Here's how the part is built. I have some questions about the finished solid (model axes, mm). Face numbers are marked on the shaded views. A direction names the side the tool comes from. Coordinates: 2 decimals unless noted, no trailing zeros. Order: outer loops, then holes, each group sorted by start corner. A loop starts at its lowest first (then second) coordinate and runs counter-clockwise, first axis right, second up. Notation, with made-up numbers: (84.5, 77.25) - (124.5, 77.25) arc R23 ccw to (124.5, 98.25) - close; hole circle Ø9 at (-20.75, 82.5). An arc over 180 degrees is marked (long way). Answer as CSV lines item,"result". Start each with the question number.
Item 1: Imagine slicing it at D-D on x = 5.5. List the corners of the cut face in (y, z) for me, and give its area (3 significant figures).
Item 2: I need wall thicknesses on line 1 (Y direction, x = 12, z = 3.75); line 2 (X direction, y = -3.5, z = -0.25); line 3 (Z direction, x = -9.5, y = 0.25). Which ranges of each line are inside material? Lowest first, please.
Item 3: On a 3-axis mill with a long thin cutter (end or side, diameter ignored), from which of +Z, -Z, +X, -X, +Y, -Y can I reach the whole of each face in a straight line? I mean the marked faces 1 and 2. Say none if no direction works.
Item 4: Imagine slicing it at B-B on x = -7. List the corners of the cut face in (y, z) for me, and give its area (3 significant figures).
Item 5: I'm going to push a flat-ended pin straight in: pin 1 (4 mm diameter, centred on x = 3.5, z = -8, fed in from -Y). Where does the tip first touch, or does it pass through?
Item 6: Imagine slicing it at A-A on z = -6. List the corners of the cut face in (x, y) for me, and give its area (3 significant figures).
Item 7: Imagine slicing it at C-C on y = -4.5. List the corners of the cut face in (x, z) for me.
from build123d import *

# Parameters (mm, degrees)
F0_W     = 44.45
F0_H     = 18.542
F1_DEPTH = 1.79912
F2_R     = 7.7851
F3_DEPTH = 3.3655


with BuildPart() as f1:
    # F0 (on Front) → F1 (new body)
    with BuildSketch(Plane.XZ):
        with Locations((-4.156615, -1.108171)):
            Rectangle(F0_W, F0_H)
    extrude(amount=F1_DEPTH)

    # F2 (on face) → F3 (join, symmetric)
    with BuildSketch(Plane.XZ.offset(1.79912)):
        with Locations((-4.23788, -0.463784)):
            Circle(F2_R)
    extrude(amount=F3_DEPTH, both=True)


solid = f1.part
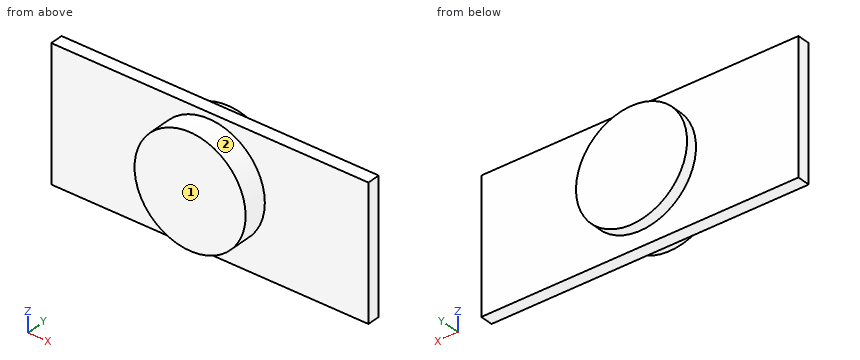
Responses:
1,outline,"(-1.8, -10.38) - (0, -10.38) - (0, 8.16) - (-1.8, 8.16) - close"
1,area,"33.4 mm^2"
2,line 1,"y = -1.8 to 0"
2,line 2,"x = -12.02 to 3.54"
2,line 3,"z = -6.2 to 5.27"
3,face 1,"+Z, -Z, +X, -X, -Y"
3,face 2,"-Y"
4,outline,"(-5.16, -7.74) - (-1.8, -7.74) - (-1.8, -10.38) - (0, -10.38) - (0, -7.74) - (1.57, -7.74) - (1.57, 6.81) - (0, 6.81) - (0, 8.16) - (-1.8, 8.16) - (-1.8, 6.81) - (-5.16, 6.81) - close"
4,area,"105 mm^2"
5,pin 1,"stops at y = -1.8"
6,outline,"(-26.38, -1.8) - (-9.71, -1.8) - (-9.71, -5.16) - (1.24, -5.16) - (1.24, -1.8) - (18.07, -1.8) - (18.07, 0) - (1.24, 0) - (1.24, 1.57) - (-9.71, 1.57) - (-9.71, 0) - (-26.38, 0) - close"
6,area,"134 mm^2"
7,outline,"circle Ø15.57 at (-4.24, -0.46)"
